Input: part model. Units: mm. Frame: model coordinates. Face numbers are marked on the shaded views. A direction names the side the tool comes from. Round coordinates to 2 decimals unless told otherwise and drop trailing zeros. Write each loop counter-clockwise with the first axis right and the second up, starting at its lowest first coordinate (ties: lowest second). Pieces come first, ordered by that corner, then holes. Notation, with made-up numbers: (-26, 28.5) -> (11, 28.5) arc R16 cw to (11, 50.5) -> close; hole circle Ø3 at (58.5, -17). An arc over 180 degrees is marked (long way). Write item = value, one per line. Start each with the question number.
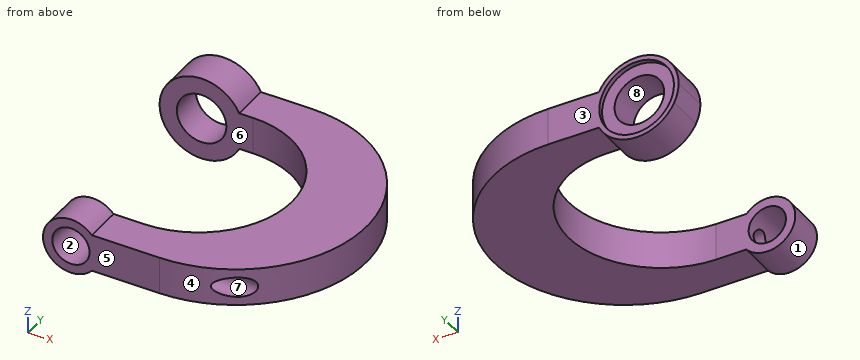
```python
from build123d import *

# Parameters (mm, degrees)
F1_DEPTH       = 44.45
F3_DEPTH       = 12.7
F5_D           = 8.4328
F5_DEPTH       = 6.35
F5_CBORE_D     = 12.7
F5_CBORE_DEPTH = 0.79375
F5_TIP         = 2.5334687141
F6_R           = 3.175
F7_DEPTH       = 25.4
F8_R           = 1.7272
F9_DEPTH       = 38.1


# Not quite as in the source:
# - a feature names something its author has since deleted; it is built from what else it names


with BuildPart() as f1:
    # F0 (on Front) → F1 (new body)
    with BuildSketch(Plane.XZ):
        with BuildLine():
            Line((-30.9068329123, 0), (0, 0))
            Line((0, 0), (0, 6.35))
            Line((0, 6.35), (-30.9068329123, 6.35))
            ThreePointArc((-30.9068329123, 6.35), (-30.3510720769, 4.8055410516), (-30.1625, 3.175))
            ThreePointArc((-30.1625, 3.175), (-30.3510720769, 1.5444589484), (-30.9068329123, 0))
        make_face()
        with BuildLine():
            ThreePointArc((-43.7056670877, 0), (-37.30625, -3.96875), (-30.9068329123, 0))
            Line((-30.9068329123, 0), (-43.7056670877, 0))
        make_face()
        with BuildLine():
            Line((-43.7056670877, 0), (-30.9068329123, 0))
            ThreePointArc((-30.9068329123, 0), (-30.3510720769, 1.5444589484), (-30.1625, 3.175))
            ThreePointArc((-30.1625, 3.175), (-30.3510720769, 4.8055410516), (-30.9068329123, 6.35))
            Line((-30.9068329123, 6.35), (-43.7056670877, 6.35))
            ThreePointArc((-43.7056670877, 6.35), (-44.2614279231, 4.8055410516), (-44.45, 3.175))
            ThreePointArc((-44.45, 3.175), (-44.2614279231, 1.5444589484), (-43.7056670877, 0))
        make_face()
        with BuildLine():
            Line((-43.7056670877, 6.35), (-30.9068329123, 6.35))
            ThreePointArc((-30.9068329123, 6.35), (-37.30625, 10.31875), (-43.7056670877, 6.35))
        make_face()
    extrude(amount=F1_DEPTH)

    # F2 (on face) → F3 (intersect, symmetric)
    with BuildSketch(Plane.XY.offset(6.35)):
        with BuildLine():
            Line((-22.225, 0), (-44.45, 0))
            Line((-44.45, 0), (-44.45, -6.35))
            Line((-44.45, -6.35), (-28.575, -6.35))
            ThreePointArc((-28.575, -6.35), (-12.7, -22.225), (-28.575, -38.1))
            Line((-28.575, -38.1), (-44.45, -38.1))
            Line((-44.45, -38.1), (-44.45, -44.45))
            Line((-44.45, -44.45), (-22.225, -44.45))
            ThreePointArc((-22.225, -44.45), (0, -22.225), (-22.225, 0))
        make_face()
    extrude(amount=F3_DEPTH, both=True, mode=Mode.INTERSECT)

    # F5
    with Locations(Plane(origin=(0, 0, 0), x_dir=(-1, 0, 0), z_dir=(0, 1, 0))):
        with Locations((37.30625, 3.175)):
            CounterBoreHole(F5_D / 2, F5_CBORE_D / 2, F5_CBORE_DEPTH, depth=F5_DEPTH)
            with Locations((0, 0, -(F5_DEPTH + F5_TIP / 2))):  # 118° drill point
                Cone(0, F5_D / 2, F5_TIP, mode=Mode.SUBTRACT)

    # F6 (on face) → F7 (cut)
    with BuildSketch(Plane.XZ.offset(44.45)):
        with BuildLine():
            ThreePointArc((-33.7564920857, 0), (-42.06875, 3.175), (-33.7564920857, 6.35))
            Line((-33.7564920857, 6.35), (-30.9068329123, 6.35))
            ThreePointArc((-30.9068329123, 6.35), (-44.45, 3.175), (-30.9068329123, 0))
            Line((-30.9068329123, 0), (-33.7564920857, 0))
        make_face()
        with Locations((-37.30625, 3.175)):
            Circle(F6_R)
    extrude(amount=-F7_DEPTH, mode=Mode.SUBTRACT)

    # F8 (on Right) → F9 (cut)
    with BuildSketch(Plane.YZ):
        with Locations((-41.275, 3.175)):
            Circle(F8_R)
    extrude(amount=-F9_DEPTH, mode=Mode.SUBTRACT)


solid = f1.part
```
1. Line query: line 1 along Y through (x, z) = (-30.5, 1); line 2 along Y through (x, z) = (-40.5, 9.5); line 3 along X through (y, z) = (-5, 4). Output: solid intervals per line, ascending.
2. Reachability of the marked faces 4, 5, 6, 7 and 8 from +Z, -Z, +X, -X, +Y, -Y: full face, straight path, thin tool, end or side. Return the list, or none.
3. Section B-B (z = 3.75). Output: boundary loops of the cut face in (x, y) (3 decimals).
4. Section C-C (x = -36). Output: boundary loops of the cut face in (y, z).
5. Section A-A (x = -15). Output: boundary loops of the cut face in (y, z) (3 decimals), then the cut area to 3 significant figures.
6. Mould query, pull axis X, two halves, no side actions, for the marked faces 1, 2 and 3. Classes: pulls with the +X half, pulls with the -X half, needs draft (parallel to the pull), parting line crosses it, or undercut.
7. Pin query (flat end, axial travel): P1, Ø2, axis at x = -9.5, z = 3, coming from the +Y side; P2, Ø1.5, axis at x = -12.5, y = -25.5, coming from the -Z side; P3, Ø6, axis at x = -13, z = 0, coming from the -Y side; P4, Ø1.5, axis at y = -26.5, z = -2, coming from the -X side. Return the tip coordinate at first contact, or that it passes through.
8. Section D-D (x = -21). Output: boundary loops of the cut face in (y, z) (3 decimals).
Check sheet entries:
q1.line_1 = -44.45 to -38.1, -6.35 to 0
q1.line_2 = -6.35 to 0
q1.line_3 = -44.4 to -41.44, -33.17 to -8.18
q2.face_4 = +Z, -Z, +X
q2.face_5 = +Z, -Z, +X, -X, -Y
q2.face_6 = +Z, -Z, -X
q2.face_7 = +X
q2.face_8 = +Y
q3.outline = (-44.427, -6.35) -> (-41.483, -6.35) -> (-41.483, -0.794) -> (-43.63, -0.794) -> (-43.63, 0) -> (-44.427, 0) -> close; (-42.034, -44.45) -> (-40.429, -44.45) -> (-40.429, -38.1) -> (-42.034, -38.1) -> close; (-34.184, -44.45) -> (-22.225, -44.45) arc R22.225 ccw to (-14.08, -42.904) -> (-34.184, -42.904) -> close; (-34.184, -39.646) -> (-8.425, -39.646) arc R22.225 ccw to (-22.225, 0) -> (-30.982, 0) -> (-30.982, -0.794) -> (-33.129, -0.794) -> (-33.129, -6.35) -> (-28.575, -6.35) arc R15.875 cw to (-28.575, -38.1) -> (-34.184, -38.1) -> close
q4.outline = (-44.45, -1.4) -> (-38.1, -1.4) -> (-38.1, 0.28) -> (-44.45, 0.28) -> close; (-44.45, 6.07) -> (-38.1, 6.07) -> (-38.1, 7.75) -> (-44.45, 7.75) -> close; (-6.35, -3.85) -> (0, -3.85) -> (0, -3.04) -> (-0.79, -3.04) -> (-0.79, -0.83) -> (-6.35, -0.83) -> close; (-6.35, 7.18) -> (-0.79, 7.18) -> (-0.79, 9.39) -> (0, 9.39) -> (0, 10.2) -> (-6.35, 10.2) -> close
q5.outline = (-43.243, 0) -> (-30.455, 0) -> (-30.455, 6.35) -> (-43.243, 6.35) -> close; (-13.995, 0) -> (-1.207, 0) -> (-1.207, 6.35) -> (-13.995, 6.35) -> close; hole circle Ø3.454 at (-41.275, 3.175)
q5.area = 153 mm2
q6.face_1 = parting line crosses it
q6.face_2 = undercut
q6.face_3 = needs draft
q7.P1 = -3.34
q7.P2 = 0
q7.P3 = -43.56
q7.P4 = through
q8.outline = (-44.416, 0) -> (-36.176, 0) -> (-36.176, 6.35) -> (-44.416, 6.35) -> close; (-8.274, 0) -> (-0.034, 0) -> (-0.034, 6.35) -> (-8.274, 6.35) -> close; hole circle Ø3.454 at (-41.275, 3.175)
